The listing builds one solid part. Answer for the finished solid, in the listing's coordinates (mm). Face numbers are marked on the shaded views. A direction names the side the tool comes from. Give positions to 0.01 mm unless a question says otherwise; leave off trailing zeros. Loops run counter-clockwise (first coordinate to the right, second up) from the corner with the lowest first, then second, coordinate; pieces in that order, holes last. Notation, with made-up numbers: M 56.5,22.5 L 67.5,22.5 A17 ccw 67.5,45.5 Z; hole C 73.5,86 d4. An arc over 180 degrees is marked long. Return JSON: item names as keys, results as strings.
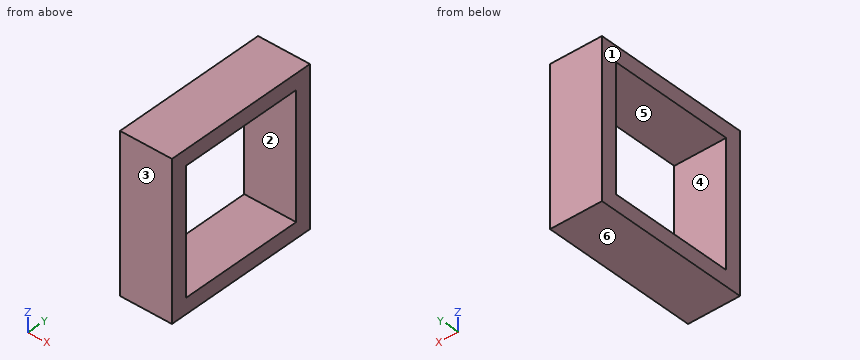
Autodesk Fusion 360 part; units mm, degrees
sketch "Sketch1" plane through (0, 0, 0) normal (1, 0, 0) x (0, 1, 0)
  line L0 (9.5131, 10.735) -> (-5.4869, 10.735)
  line L1 (-5.4869, 10.735) -> (-5.4869, -4.265)
  line L2 (-5.4869, -4.265) -> (9.5131, -4.265)
  line L3 (9.5131, -4.265) -> (9.5131, 10.735)
  line L4 (9.5131, 10.735) -> (-5.4869, -4.265) construction
  line L5 (-5.4869, 10.735) -> (9.5131, -4.265) construction
  line L6 (8.0131, -2.765) -> (-3.9869, -2.765)
  line L7 (-3.9869, -2.765) -> (-3.9869, 9.235)
  line L8 (-3.9869, 9.235) -> (8.0131, 9.235)
  line L9 (8.0131, 9.235) -> (8.0131, -2.765)
  line L10 (8.0131, -2.765) -> (-3.9869, 9.235) construction
  line L11 (-3.9869, -2.765) -> (8.0131, 9.235) construction
  point P0 (2.0131, 3.235)
  point P1 (2.0131, 3.235)
  dimension "d3" = 15
  dimension "d4" = 15
  dimension "d5" = 12
  dimension "d6" = 12
extrude "Extrude1" add sketch "Sketch1" along normal blind 5
(1) Straight lines are drawn through the part: line 1 along Z through (x, y) = (0.95, 3.5) (3 decimals); line 2 along Y through (x, z) = (2.6, 3.5). For each, find the intervals that lie inside material, in ascending order.
Values follow:
{"line 1": "-4.265 to -2.765, 9.235 to 10.735", "line 2": "-5.49 to -3.99, 8.01 to 9.51"}
(2) The part is cut by section A-A (z = 4.5). Determine the outline of the cut face in (x, y).
Values follow:
{"outline": "M 0,-5.49 L 5,-5.49 L 5,-3.99 L 0,-3.99 Z; M 0,8.01 L 5,8.01 L 5,9.51 L 0,9.51 Z"}
(3) The part is cut by section C-C (x = 2.7). Determine the outline of the cut face in (y, z) (3 decimals).
Values follow:
{"outline": "M -5.487,-4.265 L 9.513,-4.265 L 9.513,10.735 L -5.487,10.735 Z; hole M -3.987,-2.765 L 8.013,-2.765 L 8.013,9.235 L -3.987,9.235 Z"}
(4) Determine the mould class of the marked faces 1, 2, 3 and 4 for opening direction Y: released by +Y, released by -Y, zero draft, split by the parting line, or undercut.
Values follow:
{"face 1": "zero draft", "face 2": "undercut", "face 3": "released by -Y", "face 4": "undercut"}
(5) The part is cut by section B-B (y = 0.25). Determine the outline of the cut face in (x, z) (3 decimals), and give its area (3 significant figures).
Values follow:
{"outline": "M 0,-4.265 L 5,-4.265 L 5,-2.765 L 0,-2.765 Z; M 0,9.235 L 5,9.235 L 5,10.735 L 0,10.735 Z", "area": "15.0 mm²"}
(6) A tool of negligible diameter and unlimited length cuts with its end or side. For the marked faces 5 and 6, from which of +Z, -Z, +X, -X, +Y, -Y can it reach the whole face along a straight path? Write none if from no direction.
Values follow:
{"face 5": "+X, -X", "face 6": "-Z, +X, -X, +Y, -Y"}
(7) Given pin 1 (6 mm diameter, centred on y = -1.5, z = 7.5, fed in from -X), flat-ended and moving along its own axis, determine where the tip first touches the part or whether it passes through.
Values follow:
{"pin 1": "x = 0"}
